```python
from build123d import *

# Parameters (mm, degrees)
SKETCH1_R               = 44.45
SKETCH1_R_2             = 44.0436
EXTRUDE1_DEPTH          = 152.4
CUT_EXTRUDE1_START      = -152.4
CUT_EXTRUDE1_DEPTH      = 152.4
CUT_EXTRUDE2_DEPTH      = 152.4
CUT_EXTRUDE2_DEPTH_BACK = 152.4
SKETCH3_W               = 83.82
SKETCH3_H               = 76.2
CUT_EXTRUDE3_DEPTH      = 152.4
CUT_EXTRUDE3_DEPTH_BACK = 152.4
SKETCH4_W               = 28.575
SKETCH4_H               = 35.56


with BuildPart() as part:
    # Sketch1 → Extrude1 (new body)
    with BuildSketch(Plane.XY):
        with Locations(Location((0, 0, 0), (0, 0, 180))):
            Circle(SKETCH1_R)
        with Locations(Location((0, 0, 0), (0, 0, 180))):
            Circle(SKETCH1_R_2, mode=Mode.SUBTRACT)
    extrude(amount=EXTRUDE1_DEPTH)

    # Sketch2 → Cut-Extrude1 (cut)
    with BuildSketch(Plane.XY.offset(152.4).offset(CUT_EXTRUDE1_START)):
        with BuildLine():
            Line((-6.35, 43.994090512), (-6.35, 43.583439526))
            ThreePointArc((-6.35, 43.583439526), (0, 44.0436), (6.35, 43.583439526))
            Line((6.35, 43.583439526), (6.35, 43.994090512))
            ThreePointArc((6.35, 43.994090512), (0, 44.45), (-6.35, 43.994090512))
        make_face()
    extrude(amount=CUT_EXTRUDE1_DEPTH, mode=Mode.SUBTRACT)

    # Sketch3 → Cut-Extrude2 (cut, two sides: drawn at the far end of the back side and taken through both)
    with BuildSketch(Plane(origin=(0, 0, 0), x_dir=(0, 0, -1), z_dir=(1, 0, 0)).offset(-CUT_EXTRUDE2_DEPTH_BACK)):
        with Locations((-76.2, 31.75)):
            Rectangle(SKETCH3_W, SKETCH3_H)
    extrude(amount=CUT_EXTRUDE2_DEPTH + CUT_EXTRUDE2_DEPTH_BACK, mode=Mode.SUBTRACT)

    # Sketch4 → Cut-Extrude3 (cut, two sides: drawn at the far end of the back side and taken through both)
    with BuildSketch(Plane(origin=(0, 0, 0), x_dir=(0, 0, -1), z_dir=(1, 0, 0)).offset(-CUT_EXTRUDE3_DEPTH_BACK)):
        with Locations((-76.2, -24.13)):
            Rectangle(SKETCH4_W, SKETCH4_H)
    extrude(amount=CUT_EXTRUDE3_DEPTH + CUT_EXTRUDE3_DEPTH_BACK, mode=Mode.SUBTRACT)


solid = part.part
```
Design review of the part built by this model. Coordinates are the model's own, in mm. Coordinates: 2 decimals unless noted, no trailing zeros. Order: outer loops, then holes, each group sorted by start corner. A loop starts at its lowest first (then second) coordinate and runs counter-clockwise, first axis right, second up. Notation, with made-up numbers: (-35.5, -18.5) - (22.5, -18.5) arc R21 ccw to (22.5, -11.5) - close; hole circle Ø11 at (-7, 71.5). An arc over 180 degrees is marked (long way). Answer in a Markdown table with one row per item.
(1) Clearance check with flat-ended pins moving along their axes: pin 1 (1.5 mm diameter, centred on x = -13.5, z = 53, fed in from -Y); pin 2 (2 mm diameter, centred on y = -15.5, z = 115, fed in from -X); pin 3 (24.5 mm diameter, centred on x = -32.5, y = -20, fed in from -Z); pin 4 (0.5 mm diameter, centred on x = -43.5, z = 101.5, fed in from +Y). State where each tip first meets the part, or that it passes through.
Checked values:
| item | result |
|---|---|
| pin 1 | y = -42.58 |
| pin 2 | x = -42.02 |
| pin 3 | z = 0 |
| pin 4 | y = -6.35 |
(2) Consider section D-D on z = 132. State the section outline as (x, y) points.
Checked values:
| item | result |
|---|---|
| outline | (-6.35, 43.58) - (-6.35, 43.99) arc R44.45 ccw (long way) to (6.35, 43.99) - (6.35, 43.58) arc R44.04 cw (long way) to start |
(3) Consider section A-A on y = 0. State the section outline as (x, z) points.
Checked values:
| item | result |
|---|---|
| outline | (-44.45, 0) - (-44.04, 0) - (-44.04, 34.29) - (-44.45, 34.29) - close; (-44.45, 118.11) - (-44.04, 118.11) - (-44.04, 152.4) - (-44.45, 152.4) - close; (44.04, 0) - (44.45, 0) - (44.45, 34.29) - (44.04, 34.29) - close; (44.04, 118.11) - (44.45, 118.11) - (44.45, 152.4) - (44.04, 152.4) - close |
(4) Consider section B-B on x = -21.5. State the section outline as (y, z) points.
Checked values:
| item | result |
|---|---|
| outline | (-38.9, 0) - (-38.44, 0) - (-38.44, 61.91) - (-38.9, 61.91) - close; (-38.9, 90.49) - (-38.44, 90.49) - (-38.44, 152.4) - (-38.9, 152.4) - close; (38.44, 0) - (38.9, 0) - (38.9, 34.29) - (38.44, 34.29) - close; (38.44, 118.11) - (38.9, 118.11) - (38.9, 152.4) - (38.44, 152.4) - close |
(5) The part is to be moulded in two halves that separate along Z. For faces 1 (the flat face through (40, -19, 61.912)), 2 (the flat face through (-36, 25.8, 0)), 3 (the flat face through (-36, 25.8, 152.4)), say which applies: released by +Z, released by -Z, zero draft, split by the parting line, or undercut.
Checked values:
| item | result |
|---|---|
| face 1 | undercut |
| face 2 | released by -Z |
| face 3 | released by +Z |
(6) Consider section C-C on x = 10. State the section outline as (y, z) points.
Checked values:
| item | result |
|---|---|
| outline | (-43.31, 0) - (-42.89, 0) - (-42.89, 152.4) - (-43.31, 152.4) - close; (42.89, 0) - (43.31, 0) - (43.31, 34.29) - (42.89, 34.29) - close; (42.89, 118.11) - (43.31, 118.11) - (43.31, 152.4) - (42.89, 152.4) - close |
(7) Wall thickness on line 1 along Z through (x, y) = (-41, 17); line 2 along Y through (x, z) = (0, 33); line 3 along X through (y, z) = (-17, 32): over which ranges is each line inside the solid? List them lowest first. Write a range as from..to.
Checked values:
| item | result |
|---|---|
| line 1 | 0..34.29, 118.11..152.4 |
| line 2 | -44.45..-44.04 |
| line 3 | -41.07..-40.63, 40.63..41.07 |
